```python
from build123d import *

# Parameters (mm, degrees)
SKETCH1_R           = 3.96875
BOSS_EXTRUDE1_DEPTH = 1.5875


with BuildPart() as part:
    # Sketch1 → Boss-Extrude1 (new, symmetric)
    with BuildSketch(Plane(origin=(0, 0, 0), x_dir=(1, 0, 0), z_dir=(0, 1, 0))):
        Polygon((0, 303.055391585), (-200.93524919, -12.7), (200.93524919, -12.7), align=None)
        with Locations(Location((-177.8, 0, 0), (0, 0, 270))):
            Circle(SKETCH1_R, mode=Mode.SUBTRACT)
        with Locations(Location((0, 279.4, 0), (0, 0, 270))):
            Circle(SKETCH1_R, mode=Mode.SUBTRACT)
        with Locations(Location((177.8, 0, 0), (0, 0, 270))):
            Circle(SKETCH1_R, mode=Mode.SUBTRACT)
    extrude(amount=BOSS_EXTRUDE1_DEPTH, both=True)


solid = part.part
```
Source: CAD feature listing. Evaluate the final solid. Frame: model axes, mm. Give positions to 0.01 mm unless a question says otherwise; leave off trailing zeros. Loops run counter-clockwise (first coordinate to the right, second up) from the corner with the lowest first, then second, coordinate; pieces in that order, holes last. Notation, with made-up numbers: (-7.5, -17) -> (46.5, -17) arc R34 ccw to (46.5, 17) -> close; hole circle Ø11 at (53.5, -16.5). An arc over 180 degrees is marked (long way). Put each result on its own line as item: value. Start each with the question number.
1) Cut plane A-A (y = 0). Return loops of the section in (x, z), then the cut area to 3 significant figures.
2) Contact query for flat-ended pins moving along their axis: P1, Ø1, axis at y = 0.5, z = -259, coming from the -X side; P2, Ø5, axis at x = -177.8, z = 0, coming from the +Y side. Output: stop coordinate, or through.
3) Cut plane B-B (x = -118). Return loops of the section in (y, z), then the cut area to 3 significant figures.
4) Cut plane C-C (z = -144). Return loops of the section in (x, y), then the cut area to 3 significant figures.
5) Material intervals for probe 1 along X at (y, z) = (0.15, -279.4); probe 2 along X at (y, z) = (0.6, -106.5); probe 3 along X at (y, z) = (1.35, -72.5), sorted ascending.
6) Draft query along X for faces 1 (the face through (-99.06, 0.02, -147.39)), 2 (the face through (-3, -1.588, -112)), 3 (the face through (173.926, -0.022, -0.86)). Return one class per face: released by +X, released by -X, zero draft, split by the parting line, or undercut.
Results are:
1. outline: (-200.94, 12.7) -> (0, -303.06) -> (200.94, 12.7) -> close; hole circle Ø7.94 at (-177.8, 0); hole circle Ø7.94 at (0, -279.4); hole circle Ø7.94 at (177.8, 0)
1. area: 63,300 mm2
2. P1: stops at x = -28.35
2. P2: passes through
3. outline: (-1.59, -117.63) -> (1.59, -117.63) -> (1.59, 12.7) -> (-1.59, 12.7) -> close
3. area: 414 mm2
4. outline: (-101.22, -1.59) -> (101.22, -1.59) -> (101.22, 1.59) -> (-101.22, 1.59) -> close
4. area: 643 mm2
5. probe 1: x = -15.05 to -3.97, 3.97 to 15.05
5. probe 2: x = -125.08 to 125.08
5. probe 3: x = -146.72 to 146.72
6. face 1: released by -X
6. face 2: zero draft
6. face 3: undercut
